Check sheet for the modelled part. Datum: model origin and axes. Units: mm. A direction names the side the tool comes from. Coordinates: 2 decimals unless noted, no trailing zeros. Write each loop counter-clockwise with the first axis right and the second up, starting at its lowest first coordinate (ties: lowest second). Pieces come first, ordered by that corner, then holes. Notation, with made-up numbers: (-12.5, 2) -> (42.5, 2) arc R23 ccw to (42.5, 20) -> close; hole circle Ø8 at (-34, 57). An arc over 180 degrees is marked (long way). Put each result on its own line as item: value.
```python
from build123d import *

# Parameters (mm, degrees)
F0_R     = 32.5
F1_DEPTH = 3
F2_R     = 20.4
F3_DEPTH = 8
F4_R     = 19.4
F5_DEPTH = 11.001
F6_R     = 3.1
F6_R_2   = 0.551099
F7_DEPTH = 3.001


with BuildPart() as f1:
    # F0 (on Front) → F1 (new body)
    with BuildSketch(Plane.XZ):
        Circle(F0_R)
    extrude(amount=F1_DEPTH)

    # F2 (on face) → F3 (join)
    with BuildSketch(Plane.XZ.offset(3)):
        Circle(F2_R)
    extrude(amount=F3_DEPTH)

    # F4 (on face) → F5 (cut, through all)
    with BuildSketch(Plane.XZ.offset(11)):
        Circle(F4_R)
    extrude(amount=-F5_DEPTH, mode=Mode.SUBTRACT)

    # F6 (on face) → F7 (cut, through all)
    with BuildSketch(Plane.XZ.offset(3)):
        with Locations((27.5, 0)):
            Circle(F6_R)
        with Locations((-27.406738, 0)):
            Circle(F6_R)
        with Locations((0, 31.629574)):
            Circle(F6_R_2)
    extrude(amount=-F7_DEPTH, mode=Mode.SUBTRACT)


solid = f1.part
```
Q1. Depth check by flat-ended pin: P1, Ø23.5, axis at x = 0, z = 0, coming from the -Y side; P2, Ø2, axis at y = -8, z = -2.5, coming from the +X side; P3, Ø5, axis at y = -1.5, z = 18, coming from the +X side; P4, Ø2, axis at x = -18, y = -7.5, coming from the -Z side. Enter the tip coordinate at first touch or a pass-through.
Recorded:
P1: passes through
P2: stops at x = 20.34
P3: stops at x = 28.57
P4: stops at z = -11.28
Q2. Cross-section at A-A (z = 0). Record the cut outline in (x, y), plus the area to 3 significant figures.
Recorded:
outline: (-32.5, -3) -> (-30.51, -3) -> (-30.51, 0) -> (-32.5, 0) -> close; (-24.31, -3) -> (-20.4, -3) -> (-20.4, -11) -> (-19.4, -11) -> (-19.4, 0) -> (-24.31, 0) -> close; (19.4, -11) -> (20.4, -11) -> (20.4, -3) -> (24.4, -3) -> (24.4, 0) -> (19.4, 0) -> close; (30.6, -3) -> (32.5, -3) -> (32.5, 0) -> (30.6, 0) -> close
area: 57.4 mm2
Q3. Material ranges on line 1 along Z through (x, y) = (0, -1.4); line 2 along Y through (x, z) = (-28.5, 5); line 3 along Z through (x, y) = (0.5, -9), recorded low to high.
Recorded:
line 1: z = -32.5 to -19.4, 19.4 to 31.08, 32.18 to 32.5
line 2: y = -3 to 0
line 3: z = -20.39 to -19.39, 19.39 to 20.39
Q4. Cross-section at B-B (x = -11). Record the cut outline in (y, z), plus the area to 3 significant figures.
Recorded:
outline: (-11, -17.18) -> (-3, -17.18) -> (-3, -30.58) -> (0, -30.58) -> (0, -15.98) -> (-11, -15.98) -> close; (-11, 15.98) -> (0, 15.98) -> (0, 30.58) -> (-3, 30.58) -> (-3, 17.18) -> (-11, 17.18) -> close
area: 107 mm2
Q5. Tool access check on faces 1 (the cylindrical face through (18.504, -5.577, 5.827)), 2 (the flat face through (21, -3, 0)). Record the directions out of +Z, -Z, +X, -X, +Y, -Y that give a thin tool (end or side, any length) a straight path to the whole face; none if there is none.
Recorded:
face 1: +Y, -Y
face 2: -Y
Q6. Cross-section at D-D (x = 27.5). Record the cut outline in (y, z).
Recorded:
outline: (-3, -17.32) -> (0, -17.32) -> (0, -3.1) -> (-3, -3.1) -> close; (-3, 3.1) -> (0, 3.1) -> (0, 17.32) -> (-3, 17.32) -> close
Q7. Cross-section at C-C (y = -4.75). Record the cut outline in (x, z).
Recorded:
outline: circle Ø40.8 at (0, 0); hole circle Ø38.8 at (0, 0)
